from build123d import *

# Parameters (mm, degrees)
SKETCH_1_W          = 103
SKETCH_1_H          = 108
EXTRUDE_1_DEPTH     = 228
CUT_EXTRUDE_START   = -5
CUT_EXTRUDE_1_DEPTH = 218
SKETCH_3_R          = 8
CUT_EXTRUDE_2_DEPTH = 363
CUT_EXTRUDE_3_REACH = 257.947
SKETCH_4_R          = 23.5
CUT_EXTRUDE_5_DEPTH = 444
CUT_EXTRUDE_6_DEPTH = 1


with BuildPart() as part:
    # 草图1 → 凸台-拉伸1 (new body)
    with BuildSketch(Plane.XY):
        Rectangle(SKETCH_1_W, SKETCH_1_H)
    extrude(amount=-EXTRUDE_1_DEPTH)

    # 草图2 → 切除-拉伸1 (cut)
    with BuildSketch(Plane.XY.offset(CUT_EXTRUDE_START)):
        Polygon((-51.3, -49), (51.3, -49), (51.3, 49), (-0.803988537, 49), (-51.3, 49), align=None)
    extrude(amount=-CUT_EXTRUDE_1_DEPTH, mode=Mode.SUBTRACT)

    # 草图3 → 切除-拉伸2 (cut)
    with BuildSketch(Plane.XY):
        with Locations((21.4, -24.37)):
            Circle(SKETCH_3_R)
    extrude(amount=-CUT_EXTRUDE_2_DEPTH, mode=Mode.SUBTRACT)

    # 草图4 → 切除-拉伸3 (cut, up to next)
    with BuildSketch(Plane.ZY.offset(51.5), mode=Mode.PRIVATE) as cut_extrude_3_sk1:
        with Locations((-114, 5.82)):
            Circle(SKETCH_4_R)
    cut_extrude_3_tool1 = extrude(cut_extrude_3_sk1.sketch, amount=-CUT_EXTRUDE_3_REACH, mode=Mode.PRIVATE) & part.part
    add(cut_extrude_3_tool1.solids().sort_by_distance((-51.5, 5.82, -114))[0], mode=Mode.SUBTRACT)

    # 草图8 → 切除-拉伸5 (cut)
    with BuildSketch(Plane.XY):
        Polygon((0, -49), (46.5, -49), (46.5, 1), (-46.5, 1.708475641), (-46.5, -49), align=None)
    extrude(amount=-CUT_EXTRUDE_5_DEPTH, mode=Mode.SUBTRACT)

    # 草图9 → 切除-拉伸6 (cut)
    with BuildSketch(Plane(origin=(0, -49, 0), x_dir=(1, 0, 0), z_dir=(0, 1, 0))):
        Polygon((-29, 228), (11, 228), (16, 228), (16, 0), (-29, 0), align=None)
    extrude(amount=-CUT_EXTRUDE_6_DEPTH, mode=Mode.SUBTRACT)


solid = part.part
Model file for the job. Use its own axes, mm. A direction names the side the tool comes from. Coordinates: 2 decimals unless noted, no trailing zeros. Order: outer loops, then holes, each group sorted by start corner. A loop starts at its lowest first (then second) coordinate and runs counter-clockwise, first axis right, second up. Notation, with made-up numbers: M 28.5,78.5 L 74.5,78.5 A4 ccw 74.5,83.5 Z; hole C 32.25,-14 d5. An arc over 180 degrees is marked long. Return JSON: item names as keys, results as strings.
1. Tool access for faces 4 (the face through (-1, 33, -223)), 5 (the face through (-51.5, -25, -112)), 6 (the face through (46.5, -24, -2)): list every direction of +Z, -Z, +X, -X, +Y, -Y with a clear straight run to the whole face (end or side of a thin tool).
Ans:
{"face 4": "none", "face 5": "+Z, -Z, -X, +Y, -Y", "face 6": "+Z, -Z"}
2. Pull direction Y, two halves, no side cores. Call faces 1 (the face through (-1, 25, -228)), 2 (the face through (-1, 54, -112)), 3 (the face through (46.5, -24, -225)): +Y half, -Y half, draft (parallel to the pull), parting line (faces both ways), or undercut.
Ans:
{"face 1": "draft", "face 2": "+Y half", "face 3": "undercut"}
3. Drill centre lines: probe 1 along Z at (x, y) = (15, 38.5); probe 2 along Y at (x, z) = (-51.4, -114); probe 3 along Y at (x, z) = (33, -77). Where is each one in solid material? Low to high.
Ans:
{"probe 1": "-228 to -223, -5 to 0", "probe 2": "-54 to -17.68, 29.32 to 54", "probe 3": "-54 to -49, 49 to 54"}
4. Saw through at B-B (x = -33). Give the cut face in (y, z), and give its area (3 significant figures).
Ans:
{"outline": "M -54,-228 L -49,-228 L -49,0 L -54,0 Z; M 1.61,-228 L 54,-228 L 54,0 L 1.61,0 L 1.61,-5 L 49,-5 L 49,-223 L 1.61,-223 Z", "area": "2,750 mm^2"}
5. Saw through at A-A (y = -24). Give the cut face in (x, z).
Ans:
{"outline": "M -51.5,-228 L -46.5,-228 L -46.5,-223 L -51.3,-223 L -51.3,-5 L -46.5,-5 L -46.5,0 L -51.5,0 Z; M 46.5,-228 L 51.5,-228 L 51.5,0 L 46.5,0 L 46.5,-5 L 51.3,-5 L 51.3,-223 L 46.5,-223 Z"}
6. Saw through at D-D (z = -114). Give the cut face in (x, y).
Ans:
{"outline": "M -51.5,-54 L 51.5,-54 L 51.5,54 L -51.5,54 L -51.5,29.32 L -51.3,29.32 L -51.3,49 L 51.3,49 L 51.3,-49 L 16,-49 L 16,-50 L -29,-50 L -29,-49 L -51.3,-49 L -51.3,-17.68 L -51.5,-17.68 Z"}
7. Saw through at C-C (z = -55). Give the cut face in (x, y), and give its area (3 significant figures).
Ans:
{"outline": "M -51.5,-54 L 51.5,-54 L 51.5,54 L -51.5,54 Z; hole M -51.3,-49 L -29,-49 L -29,-50 L 16,-50 L 16,-49 L 51.3,-49 L 51.3,49 L -51.3,49 Z", "area": "1,020 mm^2"}
